Check sheet for the modelled part. Datum: model origin and axes. Units: mm. A direction names the side the tool comes from. Round coordinates to 2 decimals unless told otherwise and drop trailing zeros. Order: outer loops, then holes, each group sorted by start corner. A loop starts at its lowest first (then second) coordinate and runs counter-clockwise, first axis right, second up. Notation, with made-up numbers: (53, 84) -> (105, 84) arc R27 ccw to (105, 102) -> close; hole circle Ø11 at (84.5, 41.5). An arc over 180 degrees is marked (long way). Answer in a Markdown table with one row per item.
```python
from build123d import *

# Parameters (mm, degrees)
F0_R     = 6.25
F1_DEPTH = 17
F2_R     = 7.575
F3_DEPTH = 12
F5_DEPTH = 17
F6_R     = 5
F7_DEPTH = 14


with BuildPart() as f1:
    # F0 (on Front) → F1 (new body)
    with BuildSketch(Plane.XZ):
        Circle(F0_R)
    extrude(amount=F1_DEPTH)

    # F2 (on face) → F3 (join)
    with BuildSketch(Plane.XZ.offset(17)):
        Circle(F2_R)
    extrude(amount=F3_DEPTH)

    # F4 (on face) → F5 (cut, through all)
    with BuildSketch(Plane(origin=(0, 0, 0), x_dir=(-1, 0, 0), z_dir=(0, 1, 0))):
        with BuildLine():
            Line((-5.65, -2.6720778432), (-5.65, 2.6720778432))
            ThreePointArc((-5.65, 2.6720778432), (-6.25, 0), (-5.65, -2.6720778432))
        make_face()
        with BuildLine():
            ThreePointArc((6.25, 0), (6.0981554588, 1.3693063938), (5.65, 2.6720778432))
            Line((5.65, 2.6720778432), (5.65, -2.6720778432))
            ThreePointArc((5.65, -2.6720778432), (6.0981554588, -1.3693063938), (6.25, 0))
        make_face()
    extrude(amount=-F5_DEPTH, mode=Mode.SUBTRACT)

    # F6 (on face) → F7 (join)
    with BuildSketch(Plane(origin=(0, 0, 0), x_dir=(-1, 0, 0), z_dir=(0, 1, 0))):
        Circle(F6_R)
    extrude(amount=F7_DEPTH)


solid = f1.part
```
(1) Depth check by flat-ended pin: pin 1 Ø1.5 at (x, y) = (-3.5, -14) entering from -Z; pin 2 Ø1 at (x, z) = (-5.5, -1) entering from +Y; pin 3 Ø6 at (y, z) = (-12.5, 1) entering from +X. Enter the tip coordinate at first touch or a pass-through.
Solutions:
| item | result |
|---|---|
| pin 1 | z = -5.61 |
| pin 2 | y = 0 |
| pin 3 | x = 5.65 |
(2) Tool access check on faces 1 (the flat face through (2, 0, -5)), 2 (the cylindrical face through (-0.1, -8.38, -6.25)), 3 (the cylindrical face through (0.1, -8.38, 6.25)), 4 (the flat face through (-5.65, -8, 0)). Record the directions out of +Z, -Z, +X, -X, +Y, -Y that give a thin tool (end or side, any length) a straight path to the whole face; none if there is none.
Solutions:
| item | result |
|---|---|
| face 1 | +Y |
| face 2 | -Z, +Y |
| face 3 | +Z, +Y |
| face 4 | +Z, -Z, -X, +Y |
(3) Section check B-B on z = 0. Record the boundary of the cut face in (x, y) (3 decimals).
Solutions:
| item | result |
|---|---|
| outline | (-7.575, -29) -> (7.575, -29) -> (7.575, -17) -> (5.65, -17) -> (5.65, 0) -> (5, 0) -> (5, 14) -> (-5, 14) -> (-5, 0) -> (-5.65, 0) -> (-5.65, -17) -> (-7.575, -17) -> close |
(4) Section check D-D on z = 5.5. Record the boundary of the cut face in (x, y).
Solutions:
| item | result |
|---|---|
| outline | (-5.21, -29) -> (5.21, -29) -> (5.21, -17) -> (2.97, -17) -> (2.97, 0) -> (-2.97, 0) -> (-2.97, -17) -> (-5.21, -17) -> close |
(5) Section check C-C on y = 2.5. Record the boundary of the cut face in (x, z), plus the area to 3 significant figures.
Solutions:
| item | result |
|---|---|
| outline | circle Ø10 at (0, 0) |
| area | 78.5 mm^2 |
(6) Section check A-A on x = 0. Record the boundary of the cut face in (y, z) (3 decimals), plus the area to 3 significant figures.
Solutions:
| item | result |
|---|---|
| outline | (-29, -7.575) -> (-17, -7.575) -> (-17, -6.25) -> (0, -6.25) -> (0, -5) -> (14, -5) -> (14, 5) -> (0, 5) -> (0, 6.25) -> (-17, 6.25) -> (-17, 7.575) -> (-29, 7.575) -> close |
| area | 534 mm^2 |
(7) Scan lines: probe 1 along Z at (x, y) = (3.75, -12.5); probe 2 along Y at (x, z) = (6.75, -1); probe 3 along X at (y, z) = (-6.5, 2.25). Record each from-to range of solid material in increasing order. Write a range as from..to.
Solutions:
| item | result |
|---|---|
| probe 1 | -5..5 |
| probe 2 | -29..-17 |
| probe 3 | -5.65..5.65 |
